Can you work these out from the model? Positions are in its coordinate system, mm. Face numbers are marked on the shaded views. A direction names the side the tool comes from. Give positions to 0.01 mm unless a question says otherwise; leave off trailing zeros. Order: outer loops, then holes, each group sorted by start corner. A loop starts at its lowest first (then second) coordinate and runs counter-clockwise, first axis right, second up. Notation, with made-up numbers: (68, 83) - (77, 83) arc R17 cw to (77, 110) - close; hole circle Ø11 at (0, 25.25). An arc over 180 degrees is marked (long way). Return JSON: item names as keys, results as strings.
```python
from build123d import *

# Parameters (mm, degrees)
WALLS_DEPTH = 40
TABS_DEPTH  = 5
HOLES_DEPTH = 71.444664714


with BuildPart() as part:
    # Sketch1 → Walls (new body)
    with BuildSketch(Plane.XY):
        Polygon((0, 20), (-10, 20), (-10, -10), (20, -10), (20, 0), (0, 0), align=None)
    extrude(amount=-WALLS_DEPTH)

    # Sketch2 → Tabs (add)
    with BuildSketch(Plane.XY):
        with BuildLine():
            Line((20, -10), (-10, -10))
            ThreePointArc((-10, -10), (5, -43.228756555), (20, -10))
        make_face()
        with BuildLine():
            Line((-10, -10), (-10, 20))
            ThreePointArc((-10, 20), (-43.228756555, 5), (-10, -10))
        make_face()
    extrude(amount=-TABS_DEPTH)

    # Sketch3 → Holes (cut, through all)
    with BuildSketch(Plane(origin=(0, 0, -5), x_dir=(-1, 0, 0), z_dir=(0, 0, -1))):
        with BuildLine():
            Line((12.25, -5), (12.25, 15))
            ThreePointArc((12.25, 15), (15, 17.75), (17.75, 15))
            Line((17.75, 15), (17.75, 7.75))
            Line((17.75, 7.75), (35, 7.75))
            ThreePointArc((35, 7.75), (37.75, 5), (35, 2.25))
            Line((35, 2.25), (17.75, 2.25))
            Line((17.75, 2.25), (17.75, -5))
            ThreePointArc((17.75, -5), (15, -7.75), (12.25, -5))
        make_face()
        with BuildLine():
            Line((5, -17.75), (-2.25, -17.75))
            Line((-2.25, -17.75), (-2.25, -35))
            ThreePointArc((-2.25, -35), (-5, -37.75), (-7.75, -35))
            Line((-7.75, -35), (-7.75, -17.75))
            Line((-7.75, -17.75), (-15, -17.75))
            ThreePointArc((-15, -17.75), (-17.75, -15), (-15, -12.25))
            Line((-15, -12.25), (5, -12.25))
            ThreePointArc((5, -12.25), (7.75, -15), (5, -17.75))
        make_face()
    extrude(amount=-HOLES_DEPTH, mode=Mode.SUBTRACT)


solid = part.part
```
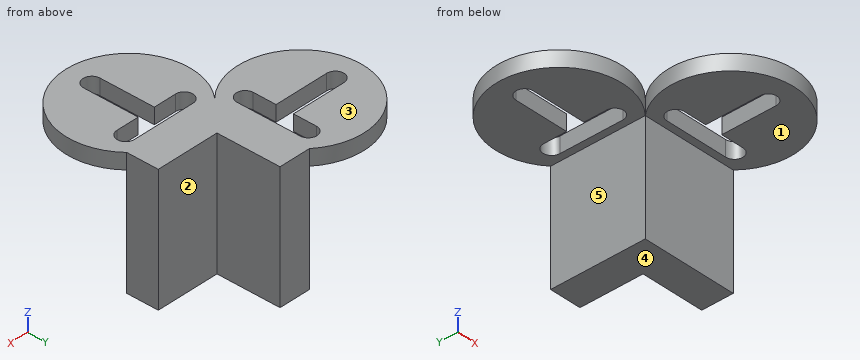
1. If I drill on L1, parallel to Y at x = -23.5, z = -3.5; L2, parallel to Y at x = 1.5, z = -5.5; L3, parallel to Z at x = -7.5, y = -37.5, over which ranges is the centre line in solid material (lowest first)? Write a range as [from, to].
Checks:
{"L1": "[-15, 2.25], [7.75, 25]", "L2": "[-10, 0]", "L3": "[-5, 0]"}
2. Suppose I cut it at C-C (z = -2.5). List the corners of the cut face in (x, y) for me.
Checks:
{"outline": "(-10, -10) arc R20 ccw (long way) to (20, -10) - (20, 0) - (0, 0) - (0, 20) - (-10, 20) arc R20 ccw (long way) to start; hole (-35, 2.25) - (-17.75, 2.25) - (-17.75, -5) arc R2.75 ccw to (-12.25, -5) - (-12.25, 15) arc R2.75 ccw to (-17.75, 15) - (-17.75, 7.75) - (-35, 7.75) arc R2.75 ccw to start; hole (-5, -17.75) - (2.25, -17.75) - (2.25, -35) arc R2.75 ccw to (7.75, -35) - (7.75, -17.75) - (15, -17.75) arc R2.75 ccw to (15, -12.25) - (-5, -12.25) arc R2.75 ccw to start"}
3. For pin 1 Ø1.5 at (x, z) = (-23, -1.5) entering from +Y; pin 2 Ø8 at (y, z) = (-3.5, -8) entering from +X; pin 3 Ø1 at (y, z) = (-5, -32) entering from -X; pin 4 Ø2.5 at (x, z) = (7.5, -1.5) entering from -Y, each with a flat end and sliding along its axis, tell me the tip position at first contact or that it passes through.
Checks:
{"pin 1": "y = 25", "pin 2": "x = 20", "pin 3": "x = -10", "pin 4": "y = -43.19"}
4. Suppose I cut it at A-A (x = 5). List the corners of the cut face in (y, z) for me.
Checks:
{"outline": "(-43.23, -5) - (-37.75, -5) - (-37.75, 0) - (-43.23, 0) - close; (-12.25, -5) - (-10, -5) - (-10, -40) - (0, -40) - (0, 0) - (-12.25, 0) - close"}
5. On a 3-axis mill with a long thin cutter (end or side, diameter ignored), from which of +Z, -Z, +X, -X, +Y, -Y can I reach the whole of each face in a straight line? I mean the marked faces 1, 2, 3, 4 and 5. Say none if no direction works.
Checks:
{"face 1": "-Z, +X, -X, -Y", "face 2": "+Z, -Z, +X, +Y", "face 3": "+Z, +X, -X, +Y, -Y", "face 4": "-Z, +X, -X, +Y, -Y", "face 5": "-Z, -X, +Y, -Y"}
6. Suppose I cut it at D-D (z = -13). List the corners of the cut face in (x, y) for me, plus the area to 3 significant figures.
Checks:
{"outline": "(-10, -10) - (20, -10) - (20, 0) - (0, 0) - (0, 20) - (-10, 20) - close", "area": "500 mm^2"}
